```python
from build123d import *

# Parameters (mm, degrees)
F0_R     = 7.5
F1_DEPTH = 3
F0_R_2   = 5.75
F2_DEPTH = 5


# Not quite as in the source:
# - a feature names something its author has since deleted; it is built from what else it names


with BuildPart() as f1:
    # F0 (on Top) → F1 (new body)
    with BuildSketch(Plane.XY):
        with BuildLine():
            Line((40, 9.5), (0, 9.5))
            ThreePointArc((0, 9.5), (-6.7175144213, 6.7175144213), (-9.5, 0))
            ThreePointArc((-9.5, 0), (-6.7175144213, -6.7175144213), (0, -9.5))
            Line((0, -9.5), (40, -9.5))
            ThreePointArc((40, -9.5), (46.7175144213, -6.7175144213), (49.5, 0))
            ThreePointArc((49.5, 0), (46.7175144213, 6.7175144213), (40, 9.5))
        make_face()
        Circle(F0_R, mode=Mode.SUBTRACT)
        with Locations((20, 0)):
            Circle(F0_R, mode=Mode.SUBTRACT)
        with Locations((40, 0)):
            Circle(F0_R, mode=Mode.SUBTRACT)
    extrude(amount=F1_DEPTH)

    # F0 (on Top) → F2 (join)
    with BuildSketch(Plane.XY):
        Circle(F0_R)
        Circle(F0_R_2, mode=Mode.SUBTRACT)
        with Locations((20, 0)):
            Circle(F0_R)
        with Locations((20, 0)):
            Circle(F0_R_2, mode=Mode.SUBTRACT)
        with Locations((40, 0)):
            Circle(F0_R)
        with Locations((40, 0)):
            Circle(F0_R_2, mode=Mode.SUBTRACT)
    extrude(amount=F2_DEPTH)


solid = f1.part
```
Can you work these out from the model? Positions are in its coordinate system, mm. A direction names the side the tool comes from. Round coordinates to 2 decimals unless told otherwise and drop trailing zeros. Loops run counter-clockwise (first coordinate to the right, second up) from the corner with the lowest first, then second, coordinate; pieces in that order, holes last. Notation, with made-up numbers: M -0.75,76.25 L 56.25,76.25 A33 cw 56.25,114.25 Z; hole C 36,68.25 d8. An arc over 180 degrees is marked long. Answer as a JSON object with one key per item and string values. Group by question number.
Q1. Will these pins go through, and if not, where does the flat tip stop? pin 1 (2 mm diameter, centred on y = 6, z = 4.5, fed in from -X); pin 2 (1.5 mm diameter, centred on x = 6.5, z = 4, fed in from +Y); pin 3 (3 mm diameter, centred on x = 23, y = 7, fed in from -Z); pin 4 (2 mm diameter, centred on y = -1.5, z = 3, fed in from +X).
Q2. Imagine slicing it at C-C, the plane x = -4. Please give me the cut outline in (y, z), then the cut area to 3 significant figures.
Q3. Imagine slicing it at D-D, the plane x = 13. Please give me the cut outline in (y, z), then the cut area to 3 significant figures.
Q4. Imagine slicing it at B-B, the plane y = 2. Please give me the cut outline in (x, z).
Q5. Please list where these lines run through material, in increasing order: L1, parallel to Y at x = 0, z = 3.5; L2, parallel to X at y = 1.25, z = 1.15; L3, parallel to Y at x = 20, z = 2.85.
Q6. We'd pull the mould along Y, two halves only. Please class faces 1 (the cylindrical face through (14.256, 0.253, 2.465)), 2 (the cylindrical face through (32.507, 0.33, 3.986)), 3 (the flat face through (-2, -6, 5)): +Y half, -Y half, draft (parallel to the pull), parting line (faces both ways), or undercut.
Q7. On a 3-axis mill with a long thin cutter (end or side, diameter ignored), from which of +Z, -Z, +X, -X, +Y, -Y can I reach the whole of each face in a straight line? I mean faces 4 (the flat face through (20, -9.5, 1)), 5 (the cylindrical face through (12.507, 0.33, 3.986)). Say none if no direction works.
Q8. Imagine slicing it at A-A, the plane x = 20. Please give me the cut outline in (y, z), then the cut area to 3 significant figures.
Findings:
{
 "1": {"pin 1": "stops at x = -5.59", "pin 2": "stops at y = 4.82", "pin 3": "stops at z = 0", "pin 4": "stops at x = 49.49"},
 "2": {"outline": "M -8.62,0 L -4.13,0 L -4.13,5 L -6.34,5 L -6.34,3 L -8.62,3 Z; M 4.13,0 L 8.62,0 L 8.62,3 L 6.34,3 L 6.34,5 L 4.13,5 Z", "area": "35.8 mm2"},
 "3": {"outline": "M -9.5,0 L 9.5,0 L 9.5,3 L 2.69,3 L 2.69,5 L -2.69,5 L -2.69,3 L -9.5,3 Z", "area": "67.8 mm2"},
 "4": {"outline": "M -9.29,0 L -5.39,0 L -5.39,5 L -7.23,5 L -7.23,3 L -9.29,3 Z; M 5.39,0 L 14.61,0 L 14.61,5 L 12.77,5 L 12.77,3 L 7.23,3 L 7.23,5 L 5.39,5 Z; M 25.39,0 L 34.61,0 L 34.61,5 L 32.77,5 L 32.77,3 L 27.23,3 L 27.23,5 L 25.39,5 Z; M 45.39,0 L 49.29,0 L 49.29,3 L 47.23,3 L 47.23,5 L 45.39,5 Z"},
 "5": {"L1": "y = -7.5 to -5.75, 5.75 to 7.5", "L2": "x = -9.42 to -5.61, 5.61 to 14.39, 25.61 to 34.39, 45.61 to 49.42", "L3": "y = -9.5 to -5.75, 5.75 to 9.5"},
 "6": {"face 1": "undercut", "face 2": "parting line", "face 3": "draft"},
 "7": {"face 4": "+Z, -Z, +X, -X, -Y", "face 5": "+Z"},
 "8": {"outline": "M -9.5,0 L -5.75,0 L -5.75,5 L -7.5,5 L -7.5,3 L -9.5,3 Z; M 5.75,0 L 9.5,0 L 9.5,3 L 7.5,3 L 7.5,5 L 5.75,5 Z", "area": "29.5 mm2"}
}
